from build123d import *

# Parameters (mm, degrees)
SKETCH1_W           = 508
SKETCH1_H           = 304.8
SKETCH1_W_2         = 50.8
SKETCH1_H_2         = 6.35
SKETCH1_W_3         = 3.175
SKETCH1_H_3         = 12.7
BOSS_EXTRUDE1_DEPTH = 3.175
SKETCH2_R           = 16.5
SKETCH2_R_2         = 1.5
CUT_EXTRUDE1_DEPTH  = 3.175
SKETCH3_R           = 1.5
CUT_EXTRUDE2_DEPTH  = 3.175


with BuildPart() as part:
    # Sketch1 → Boss-Extrude1 (new body)
    with BuildSketch(Plane.XY):
        with Locations((254, 152.4)):
            Rectangle(SKETCH1_W, SKETCH1_H)
        with Locations((50.8, -3.175)):
            Rectangle(SKETCH1_W_2, SKETCH1_H_2)
        with Locations((152.4, -3.175)):
            Rectangle(SKETCH1_W_2, SKETCH1_H_2)
        with Locations((254, -3.175)):
            Rectangle(SKETCH1_W_2, SKETCH1_H_2)
        with Locations((355.6, -3.175)):
            Rectangle(SKETCH1_W_2, SKETCH1_H_2)
        with Locations((457.2, -3.175)):
            Rectangle(SKETCH1_W_2, SKETCH1_H_2)
        with Locations((-1.5875, 19.05)):
            Rectangle(SKETCH1_W_3, SKETCH1_H_3)
        with Locations((-1.5875, 44.45)):
            Rectangle(SKETCH1_W_3, SKETCH1_H_3)
        with Locations((-1.5875, 69.85)):
            Rectangle(SKETCH1_W_3, SKETCH1_H_3)
        with Locations((-1.5875, 95.25)):
            Rectangle(SKETCH1_W_3, SKETCH1_H_3)
        with Locations((-1.5875, 120.65)):
            Rectangle(SKETCH1_W_3, SKETCH1_H_3)
        with Locations((-1.5875, 146.05)):
            Rectangle(SKETCH1_W_3, SKETCH1_H_3)
        with Locations((-1.5875, 171.45)):
            Rectangle(SKETCH1_W_3, SKETCH1_H_3)
        with Locations((-1.5875, 196.85)):
            Rectangle(SKETCH1_W_3, SKETCH1_H_3)
        with Locations((-1.5875, 222.25)):
            Rectangle(SKETCH1_W_3, SKETCH1_H_3)
        with Locations((-1.5875, 247.65)):
            Rectangle(SKETCH1_W_3, SKETCH1_H_3)
        with Locations((-1.5875, 273.05)):
            Rectangle(SKETCH1_W_3, SKETCH1_H_3)
        with Locations((-1.5875, 298.45)):
            Rectangle(SKETCH1_W_3, SKETCH1_H_3)
        with Locations((509.5875, 19.05)):
            Rectangle(SKETCH1_W_3, SKETCH1_H_3)
        with Locations((509.5875, 44.45)):
            Rectangle(SKETCH1_W_3, SKETCH1_H_3)
        with Locations((509.5875, 69.85)):
            Rectangle(SKETCH1_W_3, SKETCH1_H_3)
        with Locations((509.5875, 95.25)):
            Rectangle(SKETCH1_W_3, SKETCH1_H_3)
        with Locations((509.5875, 146.05)):
            Rectangle(SKETCH1_W_3, SKETCH1_H_3)
        with Locations((509.5875, 120.65)):
            Rectangle(SKETCH1_W_3, SKETCH1_H_3)
        with Locations((509.5875, 171.45)):
            Rectangle(SKETCH1_W_3, SKETCH1_H_3)
        with Locations((509.5875, 196.85)):
            Rectangle(SKETCH1_W_3, SKETCH1_H_3)
        with Locations((509.5875, 222.25)):
            Rectangle(SKETCH1_W_3, SKETCH1_H_3)
        with Locations((509.5875, 247.65)):
            Rectangle(SKETCH1_W_3, SKETCH1_H_3)
        with Locations((509.5875, 273.05)):
            Rectangle(SKETCH1_W_3, SKETCH1_H_3)
        with Locations((509.5875, 298.45)):
            Rectangle(SKETCH1_W_3, SKETCH1_H_3)
    extrude(amount=BOSS_EXTRUDE1_DEPTH)

    # Sketch2 → Cut-Extrude1 (cut)
    with BuildSketch(Plane.XY.offset(3.175)):
        with Locations((127, 50)):
            Circle(SKETCH2_R)
        with Locations((102, 75)):
            Circle(SKETCH2_R_2)
        with Locations((152, 75)):
            Circle(SKETCH2_R_2)
        with Locations((152, 25)):
            Circle(SKETCH2_R_2)
        with Locations((102, 25)):
            Circle(SKETCH2_R_2)
        with Locations((381, 50)):
            Circle(SKETCH2_R)
        with Locations((356, 75)):
            Circle(SKETCH2_R_2)
        with Locations((356, 25)):
            Circle(SKETCH2_R_2)
        with Locations((406, 25)):
            Circle(SKETCH2_R_2)
        with Locations((406, 75)):
            Circle(SKETCH2_R_2)
    extrude(amount=-CUT_EXTRUDE1_DEPTH, mode=Mode.SUBTRACT)

    # Sketch3 → Cut-Extrude2 (cut)
    with BuildSketch(Plane.XY.offset(3.175)):
        with Locations((15.875, 289.8)):
            Circle(SKETCH3_R)
        with Locations((15.875, 274.05)):
            Circle(SKETCH3_R)
        with Locations((492.125, 289.8)):
            Circle(SKETCH3_R)
        with Locations((492.125, 274.05)):
            Circle(SKETCH3_R)
    extrude(amount=-CUT_EXTRUDE2_DEPTH, mode=Mode.SUBTRACT)


solid = part.part
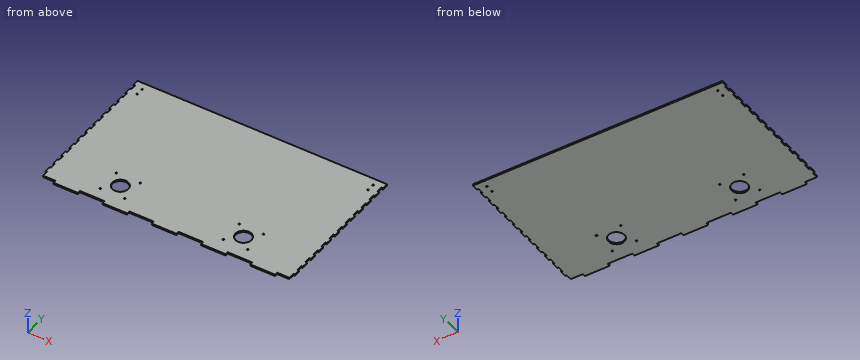
Here's how the part is built. I have some questions about the finished solid (model axes, mm). Round coordinates to 2 decimals unless told otherwise and drop trailing zeros. Write each loop counter-clockwise with the first axis right and the second up, starting at its lowest first coordinate (ties: lowest second). Pieces come first, ordered by that corner, then holes. Notation, with made-up numbers: (84.25, 13) -> (142.25, 13) arc R16 ccw to (142.25, 29) -> close; hole circle Ø9 at (-4.75, -23). An arc over 180 degrees is marked (long way). One line per item, written item: value.
1) Suppose I cut it at B-B on x = 216.5. List the corners of the cut face in (y, z) for me (3 decimals).
Filled sheet:
outline: (0, 0) -> (304.8, 0) -> (304.8, 3.175) -> (0, 3.175) -> close
2) I'm going to push flat-ended pins straight in: pin 1 Ø5 at (x, y) = (92.5, 261) entering from -Z; pin 2 Ø1 at (x, z) = (-1.5, 2) entering from -Y; pin 3 Ø1 at (y, z) = (133, 1.5) entering from -X; pin 4 Ø1 at (x, z) = (494.5, 1.5) entering from -Y. Where does each tip first touch, or does it pass through?
Filled sheet:
pin 1: stops at z = 0
pin 2: stops at y = 12.7
pin 3: stops at x = 0
pin 4: stops at y = 0
3) If I drill on line 1 (X direction, y = 75, z = 1.15) (3 decimals); line 2 (X direction, y = 59, z = 2.5); line 3 (X direction, y = 232, z = 1.15), over which ranges is the centre line in solid material (lowest first)? Write a range as [from, to].
Filled sheet:
line 1: x = [-3.175, 100.5], [103.5, 150.5], [153.5, 354.5], [357.5, 404.5], [407.5, 511.175]
line 2: x = [0, 113.17], [140.83, 367.17], [394.83, 508]
line 3: x = [0, 508]
4) Suppose I cut it at A-A on z = 1.1. Give the number of separate pieces and of enclosed holes in the cut face, plus the area to 3 significant figures.
Filled sheet:
separate pieces: 1
enclosed holes: 14
area: 156,000 mm2
